Source: three-view drawing plus pictorial views. Frame: mm from the lowest corner of the part. A direction names the side the tool comes from. Give positions to 0.01 mm unless a question says otherwise; leave off trailing zeros. Loops run counter-clockwise (first coordinate to the right, second up) from the corner with the lowest first, then second, coordinate; pieces in that order, holes last. Notation, with made-up numbers: (43.25, 68.25) - (47.25, 68.25) arc R11 cw to (47.25, 74.25) - close; hole circle Ø6 at (-33.75, -0.75). An arc over 180 degrees is marked (long way). One line per item, written item: value.
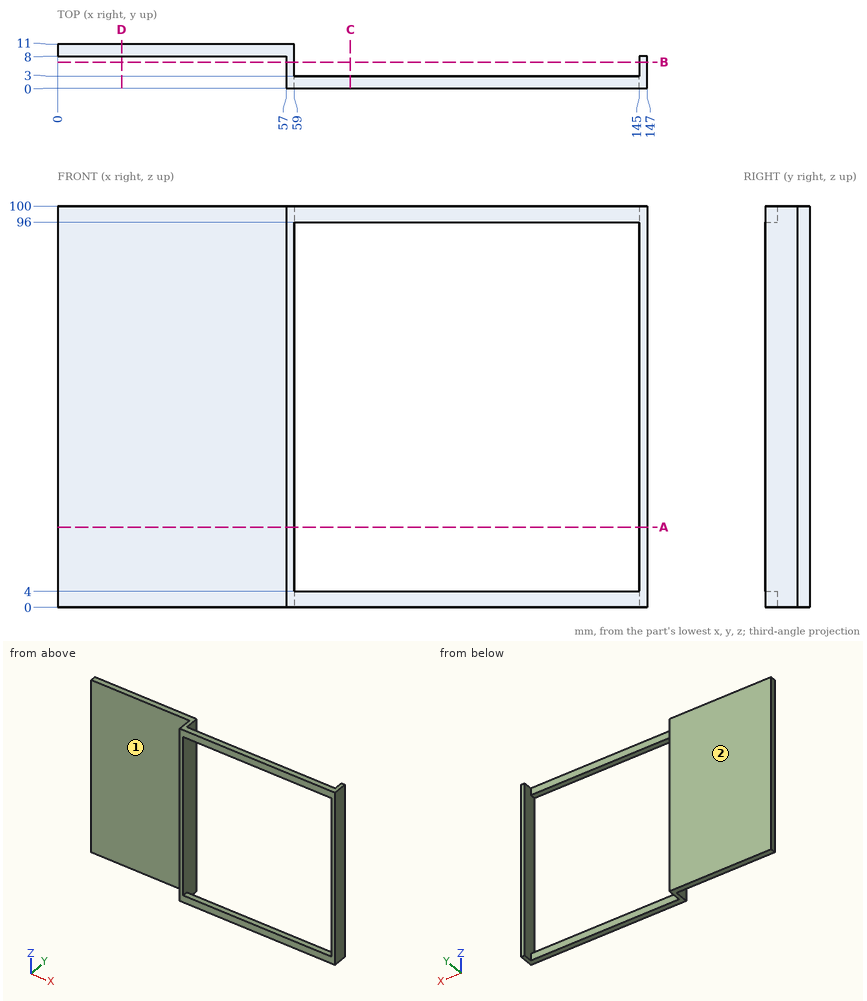
Item 1: Section A-A, the plane z = 20. Output: boundary loops of the cut face in (x, y).
Verdict:
outline: (0, 8) - (57, 8) - (57, 0) - (59, 0) - (59, 11) - (0, 11) - close; (145, 0) - (147, 0) - (147, 8) - (145, 8) - close
Item 2: Access query for the marked faces 1 and 2. Directions: +Z, -Z, +X, -X, +Y, -Y. A direction counts if a zero-diameter tool reaches every point of the face in a straight line with its end or side. Return the directions, or none.
Verdict:
face 1: +Z, -Z, -X, -Y
face 2: +Z, -Z, +X, -X, +Y
Item 3: Section B-B, the plane y = 6.5. Output: boundary loops of the cut face in (x, z).
Verdict:
outline: (57, 0) - (59, 0) - (59, 100) - (57, 100) - close; (145, 0) - (147, 0) - (147, 100) - (145, 100) - close
Item 4: Material intervals for L1, parallel to X at y = 6.5, z = 62.5; L2, parallel to X at y = 9.5, z = 71.5; L3, parallel to Y at x = 18.5, z = 67, sorted ascending.
Verdict:
L1: x = 57 to 59, 145 to 147
L2: x = 0 to 59
L3: y = 8 to 11
Item 5: Pin query (flat end, axial travel): P1, Ø6, axis at x = 23.5, z = 21.5, coming from the -Y side; P2, Ø2.5, axis at y = 2.5, z = 54, coming from the -X side; P3, Ø3, axis at x = 98.5, z = 99, coming from the +Y side. Return the tip coordinate at first contact, or that it passes through.
Verdict:
P1: stops at y = 8
P2: stops at x = 57
P3: stops at y = 3
Item 6: Section D-D, the plane x = 16. Output: boundary loops of the cut face in (y, z), and give its area (3 significant figures).
Verdict:
outline: (8, 0) - (11, 0) - (11, 100) - (8, 100) - close
area: 300 mm^2
Item 7: Section C-C, the plane x = 73. Output: boundary loops of the cut face in (y, z).
Verdict:
outline: (0, 0) - (3, 0) - (3, 4) - (0, 4) - close; (0, 96) - (3, 96) - (3, 100) - (0, 100) - close
